from build123d import *

# Parameters (mm, degrees)
SKETCH002_R       = 5
SKETCH003_W       = 14
SKETCH003_H       = 11
SKETCH004_W       = 14
SKETCH004_H       = 11
PAD_DEPTH         = 9
SKETCH006_R       = 1.75
POCKET_DEPTH      = 9.339269
POCKET_DEPTH_BACK = 9.339269
PAD001_DEPTH      = 0.2


with BuildPart() as part:
    # Sketch001 → Revolution001 (revolve)
    with BuildSketch(Plane.YZ):
        Polygon((0, 0), (3.5, 0), (4.584969, 1.879221), (3.9, 2), (3.9, 9.2), (5, 10.3), (5, 11), (0, 11), align=None)
    revolve(axis=Axis((0, 0, 0), (0, 0, 1)))

    # Sketch002 (on DatumPlane) → AdditiveLoft section 0
    with BuildSketch(Plane(origin=(0, 0, 11), x_dir=(0, -1, 0), z_dir=(0, 0, 1))):
        Circle(SKETCH002_R)
    # Sketch003 (on DatumPlane) → AdditiveLoft section 1
    with BuildSketch(Plane(origin=(0, 0, 14), x_dir=(0, -1, 0), z_dir=(0, 0, 1))):
        with Locations((0, 4.5)):
            Rectangle(SKETCH003_W, SKETCH003_H)
    # Sketch004 (on DatumPlane) → AdditiveLoft section 2
    with BuildSketch(Plane(origin=(0, 0, 24), x_dir=(0, -1, 0), z_dir=(0, 0, 1))):
        with Locations((0, 4.5)):
            Rectangle(SKETCH004_W, SKETCH004_H)
    loft(ruled=True)

    # Sketch005 → Pad (new body)
    with BuildSketch(Plane.YZ):
        Polygon((-7, 20.35), (-9.338269, 19), (-7, 17.65), (7, 17.65), (9.338269, 19), (7, 20.35), align=None)
    extrude(amount=PAD_DEPTH)

    # Sketch006 → Pocket (cut, two sides)
    with BuildSketch(Plane.XZ) as pocket_sk:
        with Locations((4.5, 19)):
            Circle(SKETCH006_R)
    extrude(amount=-POCKET_DEPTH, mode=Mode.SUBTRACT)
    extrude(pocket_sk.sketch, amount=POCKET_DEPTH_BACK, mode=Mode.SUBTRACT)

    # Sketch007 → Pad001 (join)
    with BuildSketch(Plane.XY):
        Polygon((12, 0.5), (3, 0.5), (0.5, 3), (0.5, 12), (-0.5, 12), (-0.5, 3), (-3, 0.5), (-12, 0.5), (-12, -0.5), (-3, -0.5), (-0.5, -3), (-0.5, -12), (0.5, -12), (0.5, -3), (3, -0.5), (12, -0.5), align=None)
    extrude(amount=PAD001_DEPTH)


solid = part.part
Part model, mm, in its own coordinate system. A direction names the side the tool comes from. Round coordinates to 2 decimals unless told otherwise and drop trailing zeros. Write each loop counter-clockwise with the first axis right and the second up, starting at its lowest first coordinate (ties: lowest second). Pieces come first, ordered by that corner, then holes. Notation, with made-up numbers: M 75.25,23.25 L 103.25,23.25 A32 cw 103.25,58.25 Z; hole C 18.25,42.25 d1. An arc over 180 degrees is marked long. Return JSON: item names as keys, results as strings. Group by question number.
(1) Saw through at B-B on x = -4.25. Count the separate pieces of the cut face and the enclosed holes in it, then the cut area to 3 significant figures.
(2) Drill centre lines: probe 1 along X at (y, z) = (0.25, 19); probe 2 along Y at (x, z) = (0.25, 17.5); probe 3 along Z at (x, y) = (0.25, -6.75). Where is each one in solid material? Low to high.
(3) Which spindle directions (+Z, -Z, +X, -X, +Y, -Y) get a long thin tool onto all of the face, cutting with end or side? Do faces 1 (the face through (-2.64, -2.87, 5.65)), 2 (the face through (1.293, 8.153, 18.316)), 3 (the face through (0, 8, 19)), 4 (the face through (-1, 0, 19)). Say none if no direction does.
(4) Saw through at A-A on y = -8.5. Write the cut outline in (x, z), then the cut area to 3 significant figures.
(5) Pin check, flat tips, straight feed: pin 1 Ø3 at (y, z) = (-2.5, 18.5) entering from -X; pin 2 Ø1.5 at (x, y) = (-2.5, 0.5) entering from +Z; pin 3 Ø11 at (x, z) = (4, 21) entering from -Y; pin 4 Ø5 at (x, z) = (7, 7) entering from +Y. Stop position of each tip, or through.
(6) Two-plate mould, pull along Z, no slides. Class faces 5 (the face through (1.293, -8.153, 19.684)), 6 (the face through (8, 0, 0.2)), 7 (the face through (7.659, 8.153, 18.316)): +Z half, -Z half, draft (parallel to the pull), parting line (faces both ways), or undercut.
(7) Saw through at C-C on y = 9.75. Write the cut outline in (x, z), then the cut area to 3 significant figures.
(8) Saw through at D-D on z = 5. Write the cut outline in (x, y).
Returned:
{
 "1": {"separate pieces": "3", "enclosed holes": "0", "area": "10.1 mm²"},
 "2": {"probe 1": "-1 to 2.75, 6.25 to 10", "probe 2": "-7 to 7", "probe 3": "0 to 0.2, 13.71 to 24"},
 "3": {"face 1": "none", "face 2": "+X, -X, +Y", "face 3": "+Z, -X, +Y", "face 4": "+Z, -X, +Y, -Y"},
 "4": {"outline": "M -0.5,0 L 0.5,0 L 0.5,0.2 L -0.5,0.2 Z; M 0,18.52 L 2.82,18.52 A1.75 cw 2.82,19.48 L 0,19.48 Z; M 6.18,18.52 L 9,18.52 L 9,19.48 L 6.18,19.48 A1.75 cw Z", "area": "5.57 mm²"},
 "5": {"pin 1": "x = -1", "pin 2": "z = 13.44", "pin 3": "y = -9.34", "pin 4": "through"},
 "6": {"face 5": "+Z half", "face 6": "undercut", "face 7": "-Z half"},
 "7": {"outline": "M -0.5,0 L 0.5,0 L 0.5,0.2 L -0.5,0.2 Z", "area": "0.200 mm²"},
 "8": {"outline": "C 0,0 d7.8"}
}
